The listing builds one solid part. Answer for the finished solid, in the listing's coordinates (mm). A direction names the side the tool comes from. Coordinates: 2 decimals unless noted, no trailing zeros. Loops run counter-clockwise (first coordinate to the right, second up) from the corner with the lowest first, then second, coordinate; pieces in that order, holes last. Notation, with made-up numbers: (-31, 59) - (-23, 59) arc R9 ccw to (-23, 66) - close; hole circle Ø6 at (34, 1). An arc over 180 degrees is marked (long way). Return JSON: item names as keys, results as strings. Group by question number.
1. Section A-A (y = -12.75) is taken. Write down the section's boundary in (x, z), and give its area (3 significant figures).
2. Which of the six approach directions +Z, -Z, +X, -X, +Y, -Y give full straight-line access (tool end or side, diameter ignored) to faces 1 (the face through (89.877, -9.86, 926.531)), 2 (the face through (79.74, -9.86, 470.24)), 3 (the face through (-141.38, -9.86, 968.11))?
3. Section D-D (z = 251) is taken. Write down the section's boundary in (x, y), and give its area (3 significant figures).
4. Section B-B (x = 62) is taken. Write down the section's boundary in (y, z), and give its area (3 significant figures).
5. The mould has two halves that part along X. Classify faces 4 (the face through (-157, -10, 29)), 5 (the face through (89.877, -9.86, 26.531)), 6 (the face through (79.74, -9.86, 970.24)): pulls with the +X half, pulls with the -X half, needs draft (parallel to the pull), parting line crosses it, or undercut.
6. Each of these flat-tipped pins is pushed along its axis until it touches: P1, Ø4, axis at y = -13.5, z = 379.5, coming from the +X side; P2, Ø6, axis at y = -14, z = 384.5, coming from the +X side; P3, Ø4, axis at x = -143.5, y = -3, coming from the -Z side; P4, Ø10, axis at x = 61.5, z = -5, coming from the +Y side. Where does it stop, or does it pass through?
7. Find the intervals of material crossed by line 1 along X through (y, z) = (-11, 526); line 2 along Z through (x, y) = (-113.5, -14); line 3 along Z through (x, y) = (167, -16.25), in increasing order.
8. Section C-C (z = 502.5) is taken. Write down the section's boundary in (x, y), and give its area (3 significant figures).
```python
from build123d import *

# Parameters (mm, degrees)
F1_DEPTH = 20


with BuildPart() as f1:
    # F0 (on Front) → F1 (new body)
    with BuildSketch(Plane.XZ):
        Polygon((-52.090994, 840.9694), (-52.090994, 893.185692), (-233.21149, 1045.163832), (-258.922994, 1014.522055), align=None)
        Polygon((169.029501, 1045.163832), (-12.090994, 893.185692), (-12.090994, 840.9694), (194.741005, 1014.522055), align=None)
        Polygon((-12.090994, 1140.9694), (-52.090994, 1140.9694), (-52.090994, 893.185692), (-52.090994, 840.9694), (-52.090994, 393.185692), (-52.090994, 340.9694), (-52.090994, -6.814308), (-52.090994, -59.0306), (-52.090994, -259.0306), (-12.090994, -259.0306), (-12.090994, -59.0306), (-12.090994, -6.814308), (-12.090994, 340.9694), (-12.090994, 393.185692), (-12.090994, 840.9694), (-12.090994, 893.185692), align=None)
        Polygon((-52.090994, 340.9694), (-52.090994, 393.185692), (-233.21149, 545.163832), (-258.922994, 514.522055), align=None)
        Polygon((169.029501, 545.163832), (-12.090994, 393.185692), (-12.090994, 340.9694), (194.741005, 514.522055), align=None)
        Polygon((-52.090994, -59.0306), (-52.090994, -6.814308), (-233.21149, 145.163832), (-258.922994, 114.522055), align=None)
        Polygon((169.029501, 145.163832), (-12.090994, -6.814308), (-12.090994, -59.0306), (194.741005, 114.522055), align=None)
    extrude(amount=F1_DEPTH)


solid = f1.part
```
The answers:
{
 "1": {"outline": "(-258.92, 114.52) - (-52.09, -59.03) - (-52.09, -259.03) - (-12.09, -259.03) - (-12.09, -59.03) - (194.74, 114.52) - (169.03, 145.16) - (-12.09, -6.81) - (-12.09, 340.97) - (194.74, 514.52) - (169.03, 545.16) - (-12.09, 393.19) - (-12.09, 840.97) - (194.74, 1014.52) - (169.03, 1045.16) - (-12.09, 893.19) - (-12.09, 1140.97) - (-52.09, 1140.97) - (-52.09, 893.19) - (-233.21, 1045.16) - (-258.92, 1014.52) - (-52.09, 840.97) - (-52.09, 393.19) - (-233.21, 545.16) - (-258.92, 514.52) - (-52.09, 340.97) - (-52.09, -6.81) - (-233.21, 145.16) - close", "area": "117,000 mm2"},
 "2": {"face 1": "+X, +Y, -Y", "face 2": "+Y, -Y", "face 3": "+Z, +Y, -Y"},
 "3": {"outline": "(-52.09, -20) - (-12.09, -20) - (-12.09, 0) - (-52.09, 0) - close", "area": "800 mm2"},
 "4": {"outline": "(-20, 3.14) - (0, 3.14) - (0, 55.36) - (-20, 55.36) - close; (-20, 403.14) - (0, 403.14) - (0, 455.36) - (-20, 455.36) - close; (-20, 903.14) - (0, 903.14) - (0, 955.36) - (-20, 955.36) - close", "area": "3,130 mm2"},
 "5": {"face 4": "pulls with the -X half", "face 5": "pulls with the +X half", "face 6": "undercut"},
 "6": {"P1": "stops at x = 36.21", "P2": "stops at x = 43.36", "P3": "stops at z = 15.99", "P4": "passes through"},
 "7": {"line 1": "x = -249.29 to -210.37, -52.09 to -12.09, 146.19 to 185.11", "line 2": "z = -7.5 to 44.71, 392.5 to 444.71, 892.5 to 944.71", "line 3": "z = 91.24 to 143.46, 491.24 to 543.46, 991.24 to 1043.46"},
 "8": {"outline": "(-244.6, -20) - (-182.37, -20) - (-182.37, 0) - (-244.6, 0) - close; (-52.09, -20) - (-12.09, -20) - (-12.09, 0) - (-52.09, 0) - close; (118.18, -20) - (180.41, -20) - (180.41, 0) - (118.18, 0) - close", "area": "3,290 mm2"}
}
